Geometry check sheet. Reference: the model listing, model coordinates, mm. A direction names the side the tool comes from. Round coordinates to 2 decimals unless told otherwise and drop trailing zeros. Write each loop counter-clockwise with the first axis right and the second up, starting at its lowest first coordinate (ties: lowest second). Pieces come first, ordered by that corner, then holes.
Item 1: Access from +Z, -Z, +X, -X, +Y, -Y to the whole of each face (thin tool, end or side, straight path). Record for faces 1 (the face through (793, 38.1, 0)), 2 (the face through (996, 0, 22.225)).
Item 2: Cross-section at B-B (z = 5.5). Enter the section's corners in (x, y) (1 decimal), then the cut area to 3 significant figures.
Item 3: Cross-section at C-C (y = -7.5). Enter the section's corners in (x, z) (3 decimals).
Item 4: Cross-section at D-D (x = 1688). Enter the section's corners in (y, z) (3 decimals), then the cut area to 3 significant figures.
Item 5: Cross-section at A-A (x = 1024.5). Enter the section's corners in (y, z) (3 decimals).
Item 6: Depth check by flat-ended pin: P1, Ø8, axis at x = 1699, z = -6.5, coming from the +Y side (3 decimals). Enter the tip coordinate at first touch or a pass-through.
Item 7: Scan lines: probe 1 along Y at (x, z) = (1340.5, 16); probe 2 along Z at (x, y) = (1096, 26.5) (3 decimals); probe 3 along Y at (x, z) = (536.5, -17). Record each from-to range of solid material in increasing order.
Item 8: Draft check along Y on faces 3 (the face through (1838.854, -0.178, -22.459)), 4 (the face through (1015, -34.925, 0)), 5 (the face through (1025, -38.1, 0)), 6 (the face through (996, 0, -22.225)). Enter one of: pulls with the +Y half, pulls with the -Y half, needs draft (parallel to the pull), parting line crosses it, or undercut.
Autodesk Inventor part; units mm, degrees
ref_plane "YZ Plane" through (0, 0, 0) normal (1, 0, 0) x (0, 1, 0)
ref_plane "XZ Plane" through (0, 0, 0) normal (0, 1, 0) x (-1, 0, 0)
ref_plane "XY Plane" through (0, 0, 0) normal (0, 0, 1) x (1, 0, 0)
sketch "Sketch1" plane through (0, 0, 0) normal (1, 0, 0) x (0, 1, 0)
  line L0 (-28.575, 25.4) -> (28.575, 25.4)
  line L1 (38.1, 15.875) -> (38.1, -15.875)
  line L2 (28.575, -25.4) -> (-28.575, -25.4)
  line L3 (-38.1, -15.875) -> (-38.1, 15.875)
  line L4 (-38.1, 25.4) -> (38.1, -25.4) construction
  line L5 (38.1, 25.4) -> (-38.1, -25.4) construction
  arc A0 (38.1, 15.875) -> (28.575, 25.4) centre (28.575, 15.875) ccw
  arc A1 (-28.575, 25.4) -> (-38.1, 15.875) centre (-28.575, 15.875) ccw
  arc A2 (-38.1, -15.875) -> (-28.575, -25.4) centre (-28.575, -15.875) ccw
  arc A3 (28.575, -25.4) -> (38.1, -15.875) centre (28.575, -15.875) ccw
  line L6 (34.925, -15.875) -> (34.925, 15.875)
  arc A4 (34.925, 15.875) -> (28.575, 22.225) centre (28.575, 15.875) ccw
  line L7 (28.575, 22.225) -> (-28.575, 22.225)
  arc A5 (-28.575, 22.225) -> (-34.925, 15.875) centre (-28.575, 15.875) ccw
  line L8 (-34.925, 15.875) -> (-34.925, -15.875)
  arc A6 (-34.925, -15.875) -> (-28.575, -22.225) centre (-28.575, -15.875) ccw
  line L9 (-28.575, -22.225) -> (28.575, -22.225)
  arc A7 (28.575, -22.225) -> (34.925, -15.875) centre (28.575, -15.875) ccw
  point P0 (0, 0)
  dimension "d0" = 76.2
  dimension "d1" = 50.8
  dimension "d2" = 9.525
  dimension "d3" = 3.175
extrude "Extrusion1" add sketch "Sketch1" along normal blind 2079.3737
sketch "Sketch2" plane through (0, -28.575, 25.4) normal (0, 0, 1) x (1, 0, 0)
  line L0 (0, -9.525) -> (2079.3737, -9.525)
  line L1 (0, -9.525) -> (0, 66.675)
  line L2 (0, 66.675) -> (12.0143, 66.675)
  line L3 (0, 66.675) -> (2079.3737, 66.675)
  line L4 (0, -9.525) -> (0, 0)
  line L5 (12.0143, 66.675) -> (0, -9.525)
  line L6 (2079.3737, -9.525) -> (1596.0795, 66.675)
  line L7 (1596.0795, 66.675) -> (2079.3737, 66.675)
  line L8 (2079.3737, 66.675) -> (2079.3737, -9.525)
  point P0 (0, 28.575)
  dimension "d6" = 8.96
  dimension "d7" = 8.96
extrude "Extrusion2" cut sketch "Sketch2" against normal through all contours L1 L2 L5 | L6 L3 L8
equation "\"d0\" = stockWidth"
equation "\"d1\" = stockHeight"
equation "\"d2\" = stockRad"
equation "\"d3\" = stockGuage"
equation "\"d4\" = sup2Len"
equation "\"d6\" = sup2Ang"
equation "\"d7\" = sup2Ang"
equation "\"height\" = 203.2"
equation "\"shaftDiam\" = 6.35"
equation "\"shaftSpace\" = 1.5875"
equation "\"stageSpace\" = 2.54"
equation "\"stageAngle\" = 15deg"
equation "\"stockHeight\" = 50.8"
equation "\"stockWidth\" = 76.2"
equation "\"stockRad\" = 9.525"
equation "\"stockGuage\" = 3.175"
equation "\"groundActu\" = 304.8"
equation "\"baseWidth\" = 1066.8"
equation "\"baseDepth\" = 254"
equation "\"capThickness\" = 3.175"
equation "\"sup1Len\" = 660.4"
equation "\"sup1Ang\" = 22.619865deg"
equation "\"sup2Len\" = 2079.37366"
equation "\"sup2Ang\" = 8.95995deg"
equation "\"supVertLen\" = 955.13561"
equation "\"supSideAng\" = 19.376933deg"
equation "\"supSideLen\" = 1531.12879"
equation "\"FlangeDiam\" = 12.7"
equation "\"bearingDiam\" = 9.5504"
equation "\"FlangeDepth\" = 1.5875"
equation "\"smallFilet\" = 0.39687"
equation "\"thickness\" = 12.7"
equation "\"ringDiam\" = 96.46608"
properties part number "support 2" material "Aluminum 6061"
Resolved:
1. face 1: +Z, -Z, +X, -X, +Y
1. face 2: +X, -X
2. outline: (0, -38.1) - (2079.4, -38.1) - (2059.2, -34.9) - (0.5, -34.9) - close; (11.5, 34.9) - (1616.2, 34.9) - (1596.1, 38.1) - (12, 38.1) - close
2. area: 11,600 mm2
3. outline: (4.825, -25.4) - (1885.295, -25.4) - (1885.295, -22.225) - (4.825, -22.225) - close; (4.825, 22.225) - (1885.295, 22.225) - (1885.295, 25.4) - (4.825, 25.4) - close
4. outline: (-38.1, -15.875) arc R9.525 ccw to (-28.575, -25.4) - (23.607, -25.4) - (23.607, -22.225) - (-28.575, -22.225) arc R6.35 cw to (-34.925, -15.875) - (-34.925, 15.875) arc R6.35 cw to (-28.575, 22.225) - (23.607, 22.225) - (23.607, 25.4) - (-28.575, 25.4) arc R9.525 ccw to (-38.1, 15.875) - close
4. area: 511 mm2
5. outline: (-38.1, -15.875) arc R9.525 ccw to (-28.575, -25.4) - (28.575, -25.4) arc R9.525 ccw to (38.1, -15.875) - (38.1, 15.875) arc R9.525 ccw to (28.575, 25.4) - (-28.575, 25.4) arc R9.525 ccw to (-38.1, 15.875) - close; hole (-34.925, -15.875) arc R6.35 ccw to (-28.575, -22.225) - (28.575, -22.225) arc R6.35 ccw to (34.925, -15.875) - (34.925, 15.875) arc R6.35 ccw to (28.575, 22.225) - (-28.575, 22.225) arc R6.35 ccw to (-34.925, 15.875) - close
6. P1: stops at y = -34.925
7. probe 1: y = -38.1 to -34.92, 34.92 to 38.1
7. probe 2: z = -25.4 to -22.225, 22.225 to 25.4
7. probe 3: y = -38.03 to -34.82, 34.82 to 38.03
8. face 3: pulls with the +Y half
8. face 4: undercut
8. face 5: pulls with the -Y half
8. face 6: undercut
